Input: part model. Units: mm. Frame: model coordinates. A direction names the side the tool comes from. Coordinates: 2 decimals unless noted, no trailing zeros. Order: outer loops, then holes, each group sorted by start corner. A loop starts at its lowest first (then second) coordinate and runs counter-clockwise, first axis right, second up. Notation, with made-up numbers: M -33.75,88 L -24.75,88 A19 cw -24.75,111 Z; hole C -22.5,47.25 d2. An arc over 180 degrees is marked long. One line per item, written item: value.
Autodesk Inventor part; units mm, degrees
ref_plane "YZ Plane" through (0, 0, 0) normal (1, 0, 0) x (0, 1, 0)
ref_plane "XZ Plane" through (0, 0, 0) normal (0, 1, 0) x (-1, 0, 0)
ref_plane "XY Plane" through (0, 0, 0) normal (0, 0, 1) x (1, 0, 0)
sketch "Sketch1" plane through (0, 0, 0) normal (0, 1, 0) x (-1, 0, 0)
  line L0 (4.9223, 0.8124) -> (4.9223, -5.2521)
  line L1 (5.9223, -6.2521) -> (6.9223, -6.2521)
  line L2 (6.9223, -6.2521) -> (6.9223, 4.8364)
  line L3 (6.9223, 4.8364) -> (3.5067, 4.8364)
  arc A0 (3.5067, 4.8364) -> (0.6365, -5.8307) centre (4.4005, -1.1238) ccw
  arc A1 (4.0891, 2.8364) -> (2.4729, -5.0213) centre (4, -1.2403) ccw
  arc A2 (2.9716, -5.4611) -> (2.4729, -5.0213) centre (2.0984, -5.9485) ccw
  arc A3 (4.9223, -5.2521) -> (5.9223, -6.2521) centre (5.9223, -5.2521) ccw
  line L4 (4.9223, 0.8124) -> (4.9223, 1.8364)
  line L5 (3.9223, 2.8364) -> (4.0891, 2.8364)
  arc A4 (4.9223, 1.8364) -> (3.9223, 2.8364) centre (3.9223, 1.8364) ccw
  line L6 (0.8547, -5.917) -> (2.5906, -6.0548)
  arc A5 (2.5906, -6.0548) -> (2.9716, -5.4611) centre (2.6223, -5.656) ccw
  arc A6 (0.6365, -5.8307) -> (0.8547, -5.917) centre (0.8864, -5.5183) ccw
  point P0 (0, 0)
  point P1 (4.9223, -6.2521)
  point P2 (2.9653, -6.9772)
  point P3 (2.8675, -5.1576)
  point P4 (3.0877, -6.0942)
  point P5 (0.7347, -5.9075)
  dimension "d1" = 2
  dimension "d5" = 1
  dimension "d7" = 5
  dimension "d8" = 1
  dimension "d9" = 2
  dimension "d10" = 1
  dimension "d13" = 0.4
  dimension "d14" = 2.3
extrude "Extrusion1" add sketch "Sketch1" along normal blind 6
properties part number "cable hook 5mm-2mm opening"
(1) First-contact query: pin 1 (2 mm diameter, centred on y = 1, z = 2.5, fed in from +X). Flat tip, straight axial feed; report the tip coordinate or a pass-through.
Data:
pin 1: stops at x = 1.03
(2) Cut plane B-B on x = -0.25. Output: boundary loops of the cut face in (y, z).
Data:
outline: M 0,-5.49 L 6,-5.49 L 6,-2.84 L 0,-2.84 Z; M 0,0.36 L 6,0.36 L 6,3.25 L 0,3.25 Z
(3) Ray query, line 1 (X direction, y = 1.9, z = -5.5); line 2 (X direction, y = 5.2, z = -5); line 3 (Z direction, x = -2.75, y = 2.95). Return the intervals inside material, ascending. Write a range as from..to.
Data:
line 1: x = -6.92..-4.95, -2.99..-0.26
line 2: x = -6.92..-4.92, -2.42..0.21
line 3: z = -6.04..-5.19, 2.64..4.67
(4) Cut plane A-A on z = 0.5. Output: boundary loops of the cut face in (x, y).
Data:
outline: M -6.92,0 L -4.92,0 L -4.92,6 L -6.92,6 Z; M -0.31,0 L 1.4,0 L 1.4,6 L -0.31,6 Z
(5) Cut plane D-D on x = -4.75. Output: boundary loops of the cut face in (y, z), plus the area to 3 significant figures.
Data:
outline: M 0,2.4 L 6,2.4 L 6,4.84 L 0,4.84 Z
area: 14.6 mm2
(6) Cut plane C-C on y = 2. Output: boundary loops of the cut face in (x, z), plus the area to 3 significant figures.
Data:
outline: M -6.92,-6.25 L -5.92,-6.25 A1 ccw -4.92,-5.25 L -4.92,1.84 A1 cw -3.92,2.84 A4.08 cw -2.47,-5.02 A1 ccw -2.97,-5.46 A0.4 ccw -2.59,-6.05 L -0.85,-5.92 A0.4 ccw -0.64,-5.83 A6.03 ccw -3.51,4.84 L -6.92,4.84 Z
area: 47.0 mm2
(7) Access query for faces 1 (the cylindrical face through (-5.223, 2.958, -5.967)), 2 (the flat face through (-6.4, 3, -6.252)). Directions: +Z, -Z, +X, -X, +Y, -Y. A direction counts if a zero-diameter tool reaches every point of the face in a straight line with its end or side. Return the directions, or none.
Data:
face 1: -Z, +Y, -Y
face 2: -Z, +X, -X, +Y, -Y
(8) Draft query along Z for faces 3 (the cylindrical face through (0.023, 2.958, -0.578)), 4 (the flat face through (-6.922, 3, -1)), 5 (the cylindrical face through (-4.62, 2.96, 2.55)). Return one class per face: released by +Z, released by -Z, zero draft, split by the parting line, or undercut.
Data:
face 3: undercut
face 4: zero draft
face 5: released by -Z
